Source: CAD feature listing. Evaluate the final solid. Frame: model axes, mm. A direction names the side the tool comes from. Round coordinates to 2 decimals unless told otherwise and drop trailing zeros. Order: outer loops, then holes, each group sorted by start corner. A loop starts at its lowest first (then second) coordinate and runs counter-clockwise, first axis right, second up. Notation, with made-up numbers: (31, 5.25) -> (39, 5.25) arc R12 cw to (39, 12.25) -> close; hole circle Ø10 at (62.5, 40.5). An arc over 180 degrees is marked (long way). Write item = value, one per line. Start each with the question number.
(1) Ray query, line 1 (Y direction, x = 0, z = 0.6) (3 decimals); line 2 (Y direction, x = 0, z = -1.8) (3 decimals); line 3 (X direction, y = 3, z = -1.25) (3 decimals). Return the intervals inside material, ascending.
(2) Reachability of faces 4 (the face through (0.03, 5.92, -2.13)), 5 (the face through (1.765, 7.601, -0.014)), 6 (the face through (-1.734, 7.57, -0.014)) from +Z, -Z, +X, -X, +Y, -Y: full face, straight path, thin tool, end or side. Return the list, or none.
(3) Cut plane C-C on x = 1.55. Return the cut outline in (y, z).
(4) Cut plane D-D on y = 3. Return the cut outline in (x, z) (3 decimals), then the cut area to 3 significant figures.
(5) Draft query along Y for faces 1 (the face through (-1.734, 11.43, 0.033)), 2 (the face through (-0.033, 5.916, 2.134)), 3 (the face through (0, 5, 0)). Return one class per face: released by +Y, released by -Y, zero draft, split by the parting line, or undercut.
(6) Cut plane A-A on z = -0.3. Return the cut outline in (x, y) (3 decimals).
(7) Cut plane B-B on x = -0.1. Return the cut outline in (y, z), then the cut area to 3 significant figures.
(8) Contact query for flat-ended pins moving along their axis: pin 1 Ø1.2 at (x, y) = (0, 8) entering from +Z; pin 2 Ø1.9 at (x, y) = (0, 3) entering from -Z. Output: stop coordinate, or through.
from build123d import *

# Parameters (mm, degrees)
BOSS_EXTRUDE1_DEPTH     = 10
BOSS_EXTRUDE2_DEPTH     = 2
SKETCH4_W               = 2
SKETCH4_H               = 2
CUT_EXTRUDE1_DEPTH      = 4.67
FILLET1_R               = 2
SKETCH6_R               = 1.165
CUT_EXTRUDE2_DEPTH      = 3.335
CUT_EXTRUDE2_DEPTH_BACK = 3.335


with BuildPart() as part:
    # Sketch2 → Boss-Extrude1 (new body)
    with BuildSketch(Plane(origin=(0, 0, 0), x_dir=(1, 0, 0), z_dir=(0, 1, 0))):
        Polygon((-2.335, -2.335), (-2.335, 2.335), (2.335, 1.926427941), (2.335, -1.926427941), align=None)
    extrude(amount=BOSS_EXTRUDE1_DEPTH)

    # Sketch3 → Boss-Extrude2 (add)
    with BuildSketch(Plane(origin=(0, 10, 0), x_dir=(1, 0, 0), z_dir=(0, 1, 0))):
        Polygon((2.335, -1.926427941), (2.335, 1.926427941), (-2.335, 2.335), (-2.335, -2.335), align=None)
    extrude(amount=BOSS_EXTRUDE2_DEPTH)

    # Sketch4 → Cut-Extrude1 (cut)
    with BuildSketch(Plane(origin=(2.335, 0, 0), x_dir=(0, 0, -1), z_dir=(1, 0, 0))):
        with Locations((0, 6)):
            Rectangle(SKETCH4_W, SKETCH4_H)
    extrude(amount=-CUT_EXTRUDE1_DEPTH, mode=Mode.SUBTRACT)

    # Fillet1
    fillet1_edges = [part.edges().sort_by_distance(p)[0] for p in [
        (2.335, 12, 0),
        (-2.335, 12, 0),
        (2.335, 7, 0),
        (-2.335, 7, 0),
    ]]
    fillet(fillet1_edges, radius=FILLET1_R)

    # Sketch6 → Cut-Extrude2 (cut, two sides)
    with BuildSketch(Plane.XY) as cut_extrude2_sk:
        with Locations((0, 3)):
            Circle(SKETCH6_R)
    extrude(amount=CUT_EXTRUDE2_DEPTH, mode=Mode.SUBTRACT)
    extrude(cut_extrude2_sk.sketch, amount=-CUT_EXTRUDE2_DEPTH_BACK, mode=Mode.SUBTRACT)


solid = part.part
Evaluation:
q1.line_1 = 0 to 1.835, 4.165 to 5, 7 to 12
q1.line_2 = 0 to 1.835, 4.165 to 12
q1.line_3 = -2.335 to -1.165, 1.165 to 2.335
q2.face_4 = -Z, +X, +Y, -Y
q2.face_5 = +X
q2.face_6 = -X
q3.outline = (0, -2) -> (11.59, -2) -> (11.59, 2) -> (0, 2) -> close; hole (5, -1) -> (7.41, -1) -> (7.41, 1) -> (5, 1) -> close
q4.outline = (-2.335, -2.335) -> (-1.165, -2.233) -> (-1.165, 2.233) -> (-2.335, 2.335) -> close; (1.165, -2.029) -> (2.335, -1.926) -> (2.335, 1.926) -> (1.165, 2.029) -> close
q4.area = 9.97 mm^2
q5.face_1 = released by +Y
q5.face_2 = zero draft
q5.face_3 = undercut
q6.outline = (-2.335, 0) -> (2.335, 0) -> (2.335, 5) -> (-2.335, 5) -> close; (-2.335, 9) arc R2 ccw to (-0.335, 7) -> (0.335, 7) arc R2 ccw to (2.335, 9) -> (2.335, 10) arc R2 ccw to (0.335, 12) -> (-0.335, 12) arc R2 ccw to (-2.335, 10) -> close; hole circle Ø2.33 at (0, 3)
q7.outline = (0, -2.14) -> (1.84, -2.14) -> (1.84, 2.14) -> (0, 2.14) -> close; (4.16, -2.14) -> (12, -2.14) -> (12, 2.14) -> (4.16, 2.14) -> close; hole (5, -1) -> (7, -1) -> (7, 1) -> (5, 1) -> close
q7.area = 37.4 mm^2
q8.pin_1 = 2.18
q8.pin_2 = through
